```python
from build123d import *
from build123d.topology import SkipClean

# Parameters (mm, degrees)
BOSS_EXTRUDE4_DEPTH    = 1.5
FILLET1_R              = 2
BOSS_EXTRUDE5_DEPTH    = 8.75
FILLET4_R              = 10
FILLET5_R              = 10
FILLET4_OF_MIRROR2_R   = 10
FILLET5_OF_MIRROR2_R   = 10
CUT_EXTRUDE2_START     = -26.018483
CUT_EXTRUDE2_OUTLINE_W = 14.5
CUT_EXTRUDE2_OUTLINE_H = 14
CUT_EXTRUDE2_DEPTH     = 24.018483
CUT_EXTRUDE3_DEPTH     = 48.40824


# Read off the part's stored shape, not the designer's step: Cut-Extrude2
with BuildPart() as part:
    # Sketch1 → Boss-Extrude4 (new body)
    with BuildSketch(Plane(origin=(0, 0, 0), x_dir=(1, 0, 0), z_dir=(0, 1, 0))):
        with BuildLine():
            Line((-7.070184, 12.5), (-8.75, 12.5))
            Line((-8.75, 12.5), (-8.75, -12.5))
            Line((-8.75, -12.5), (8.75, -12.5))
            Line((8.75, -12.5), (8.75, 12.5))
            Line((8.75, 12.5), (7.070184, 12.5))
            ThreePointArc((7.070184, 12.5), (0, 10.35), (-7.070184, 12.5))
        make_face()
    extrude(amount=BOSS_EXTRUDE4_DEPTH)

    # Fillet1
    # the kernel refuses this fillet: 2 mm, written as the material it takes off along each edge
    with BuildSketch(Plane(origin=(-8.75, -4.935511, -12.5), x_dir=(1, 0, 0), z_dir=(0, 1, 0))) as fillet1_piece_1:
        with BuildLine():
            CenterArc((2, -1.974204), FILLET1_R, 99.212233, 80.787767)
            Line((0, -1.974204), (-0.04, -1.974204))
            Line((-0.04, -1.974204), (-0.04, 0))
            Line((-0.04, 0), (0, 0.04))
            ThreePointArc((0, 0.04), (0.839908, 0.04), (1.673412, 0.039484))
            Line((1.673412, 0.039484), (1.679816, 0))
        make_face()
    extrude(amount=11.371021, mode=Mode.SUBTRACT)
    with BuildSketch(Plane(origin=(8.75, -4.935511, -12.5), x_dir=(0, 0, 1), z_dir=(0, 1, 0))) as fillet1_piece_2:
        with BuildLine():
            CenterArc((1.974204, -2), FILLET1_R, 90, 80.787767)
            Line((0, -1.679816), (-0.039484, -1.673412))
            ThreePointArc((-0.039484, -1.673412), (-0.04, -0.839908), (-0.04, 0))
            Line((-0.04, 0), (0, 0.04))
            Line((0, 0.04), (1.974204, 0.04))
            Line((1.974204, 0.04), (1.974204, 0))
        make_face()
    extrude(amount=11.371021, mode=Mode.SUBTRACT)
    with BuildSketch(Plane(origin=(-8.75, -5, 12.5), x_dir=(0, 0, -1), z_dir=(0, 1, 0)), Plane(origin=(8.75, -5, 12.5), x_dir=(-1, 0, 0), z_dir=(0, 1, 0))) as fillet1_piece_3:
        with BuildLine():
            CenterArc((FILLET1_R, -FILLET1_R), FILLET1_R, 90, 90)
            Line((0, -FILLET1_R), (-FILLET1_R * 0.02, -FILLET1_R))
            Line((-FILLET1_R * 0.02, -FILLET1_R), (-FILLET1_R * 0.02, FILLET1_R * 0.02))
            Line((-FILLET1_R * 0.02, FILLET1_R * 0.02), (FILLET1_R, FILLET1_R * 0.02))
            Line((FILLET1_R, FILLET1_R * 0.02), (FILLET1_R, 0))
        make_face()
    extrude(amount=11.5, mode=Mode.SUBTRACT)

    # Sketch2 → Boss-Extrude5 (add)
    with BuildSketch(Plane(origin=(8.75, 0, 0), x_dir=(0, 0, -1), z_dir=(1, 0, 0))):
        with BuildLine():
            Line((-10.5, 1.5), (11.817003, 19.5))
            Line((11.817003, 19.5), (29.817003, 19.5))
            Line((29.817003, 19.5), (29.817003, 15.5))
            Line((29.817003, 15.5), (13.518483, 15.5))
            Line((13.518483, 15.5), (1.89958, 6.128658))
            ThreePointArc((1.89958, 6.128658), (1.912979, 3.332502), (4.024993, 1.5))
            Line((4.024993, 1.5), (-1.921972, 1.5))
            Line((-1.921972, 1.5), (-10.5, 1.5))
        make_face()
    boss_extrude5 = extrude(amount=-BOSS_EXTRUDE5_DEPTH)

    # Fillet4
    # the kernel refuses this fillet: 10 mm, written as the material it takes off along each edge
    with BuildSketch(Plane(origin=(28.75, 19.5, -29.817003), x_dir=(0, 0, 1), z_dir=(-1, 0, 0))) as fillet4_piece_1:
        with BuildLine():
            CenterArc((8, -10), FILLET4_R, 90, 53.130102)
            Line((0, -4), (-0.16, -3.88))
            ThreePointArc((-0.16, -3.88), (-0.2, -2), (-0.2, 0))
            Line((-0.2, 0), (0, 0.2))
            Line((0, 0.2), (8, 0.2))
            Line((8, 0.2), (8, 0))
        make_face()
    extrude(amount=48.75, mode=Mode.SUBTRACT)

    # Fillet5
    fillet5_edges = [part.edges().sort_by_distance(p)[0] for p in [
        (4.375, 19.5, -11.817003),
    ]]
    fillet(fillet5_edges, radius=FILLET5_R)

    # Mirror2: Boss-Extrude5 across plane
    add(boss_extrude5.mirror(Plane(origin=(0, 0, 0), x_dir=(0, 0, 1), z_dir=(1, 0, 0))))

    # Fillet4 of Mirror2
    # the kernel refuses this fillet: 10 mm, written as the material it takes off along each edge
    with BuildSketch(Plane(origin=(-28.75, 19.5, -29.817003), x_dir=(0, -1, 0), z_dir=(1, 0, 0))) as fillet4_of_mirror2_piece_1:
        with BuildLine():
            CenterArc((10, -8), FILLET4_OF_MIRROR2_R, 126.869898, 53.130102)
            Line((0, -8), (-0.2, -8))
            Line((-0.2, -8), (-0.2, 0))
            Line((-0.2, 0), (0, 0.2))
            ThreePointArc((0, 0.2), (2, 0.2), (3.88, 0.16))
            Line((3.88, 0.16), (4, 0))
        make_face()
    extrude(amount=48.75, mode=Mode.SUBTRACT)

    # Fillet5 of Mirror2
    fillet5_of_mirror2_edges = [part.edges().sort_by_distance(p)[0] for p in [
        (-4.375, 19.5, -11.817003),
    ]]
    fillet(fillet5_of_mirror2_edges, radius=FILLET5_OF_MIRROR2_R)

    # Cut-Extrude2 outline → Cut-Extrude2 (cut)
    with SkipClean():  # the faces are left unmerged after this step: merging them gives an invalid solid
        with BuildSketch(Plane.XY.offset(12.5).offset(CUT_EXTRUDE2_START)):
            with Locations((0, 8.5)):
                Rectangle(CUT_EXTRUDE2_OUTLINE_W, CUT_EXTRUDE2_OUTLINE_H)
        extrude(amount=CUT_EXTRUDE2_DEPTH, mode=Mode.SUBTRACT)

    # Sketch5 → Cut-Extrude3 (cut, through all)
    with SkipClean():  # the faces are left unmerged after this step: merging them gives an invalid solid
        with BuildSketch(Plane.XY.offset(12.5)):
            with BuildLine():
                Line((-7.25, 15.5), (7.25, 15.5))
                add(Edge.make_bspline(
                    [(7.25, 15.5), (0, 16.542635), (-7.25, 15.5)],
                    knots=[0, 0, 0, 1, 1, 1], degree=2))
            make_face()
        extrude(amount=-CUT_EXTRUDE3_DEPTH, mode=Mode.SUBTRACT)


solid = part.part
```
Work out the finished part from the listing and answer in its coordinate system (mm). A direction names the side the tool comes from. Give positions to 0.01 mm unless a question says otherwise; leave off trailing zeros. Write each loop counter-clockwise with the first axis right and the second up, starting at its lowest first coordinate (ties: lowest second). Pieces come first, ordered by that corner, then holes. Notation, with made-up numbers: (66.5, -30.75) -> (82.5, -30.75) arc R11 cw to (82.5, -13.75) -> close; hole circle Ø6 at (-37.5, 80). An arc over 180 degrees is marked (long way). Write each question's results on one line, items separated by ' | '.
1. Determine the mould class of faces 1 (the cylindrical face through (-8.26, 0.74, -11.84)), 2 (the flat face through (8, 15.5, -22)), 3 (the flat face through (7.25, 7, -2)) for opening direction X: +X half, -X half, draft (parallel to the pull), parting line (faces both ways), or undercut.
Data:
face 1: -X half | face 2: draft | face 3: undercut
2. Find section A-A on y = 11. Determine the outline of the cut face in (x, z).
Data:
outline: (-8.75, -7.94) -> (-7.25, -7.94) -> (-7.25, -1.28) -> (-8.75, -1.28) -> close; (7.25, -7.94) -> (8.75, -7.94) -> (8.75, -1.28) -> (7.25, -1.28) -> close
3. Find section B-B on z = 0. Determine the outline of the cut face in (x, y).
Data:
outline: (-8.75, 0) -> (8.75, 0) -> (8.75, 9.97) -> (7.25, 9.97) -> (7.25, 1.5) -> (-7.25, 1.5) -> (-7.25, 9.97) -> (-8.75, 9.97) -> close
4. Straight lines are drawn through the part: L1, parallel to X at y = 3, z = 1; L2, parallel to Y at x = -1.5, z = 1; L3, parallel to Z at x = 2, y = 17.5. For each, find the intervals that lie inside material, in ascending order.
Data:
L1: -8.75 to -7.25, 7.25 to 8.75 | L2: 0 to 1.5 | L3: -27.82 to -9.35
5. Find section C-C on y = 4.75. Determine the outline of the cut face in (x, z).
Data:
outline: (-8.75, -1.6) -> (-7.25, -1.6) -> (-7.25, 6.47) -> (-8.75, 6.47) -> close; (7.25, -1.6) -> (8.75, -1.6) -> (8.75, 6.47) -> (7.25, 6.47) -> close
6. Find section D-D on z = -7.5. Give the number of separate pieces and of enclosed holes in the cut face, and give its area (3 significant figures).
Data:
separate pieces: 3 | enclosed holes: 0 | area: 44.8 mm^2
7. A tool of negligible diameter and unlimited length cuts with its end or side. For faces 4 (the flat face through (7.99, 10.88, -7.79)), 5 (the flat face through (-7.25, 7, -2)), 6 (the cylindrical face through (-8.18, 0.74, 11.9)), 7 (the cylindrical face through (0.1, 0.74, -10.35)), from which of +Z, -Z, +X, -X, +Y, -Y can it reach the whole face along a straight path? Write none if from no direction.
Data:
face 4: -Z, +X, -X | face 5: +Z, -Z | face 6: +Z, -X, +Y, -Y | face 7: -Z, -Y
8. Each of these flat-tipped pins is pushed along its axis until it touches: pin 1 Ø2 at (x, z) = (-1.5, -8) entering from +Y; pin 2 Ø1.5 at (x, z) = (2.5, -20.5) entering from -Y; pin 3 Ø1.6 at (x, z) = (-7.5, -19) entering from -Y. Where does it stop, or does it pass through?
Data:
pin 1: y = 17.23 | pin 2: y = 15.92 | pin 3: y = 15.5
